Build history of the part. All positions in model axes, mm. Face numbers are marked on the shaded views. A direction names the side the tool comes from. Give positions to 0.01 mm unless a question says otherwise; leave off trailing zeros. Write each loop counter-clockwise with the first axis right and the second up, starting at its lowest first coordinate (ties: lowest second). Pieces come first, ordered by that corner, then holes. Notation, with made-up numbers: (36, -31) -> (41, -31) arc R22 ccw to (41, 6) -> close; hole circle Ø7 at (26.5, 88.25). An arc over 180 degrees is marked (long way). Write item = value, one per line. Start each with the question number.
Q1. Tool access for the marked faces 1 and 2: list every direction of +Z, -Z, +X, -X, +Y, -Y with a clear straight run to the whole face (end or side of a thin tool).
Q2. Wall check: line 1 (X direction, y = 10, z = 3); line 2 (X direction, y = 44, z = 18.5); line 3 (Y direction, x = 140, z = -1.75). Give the ranges that are in metal, low to high.
Q3. Saw through at A-A, the plane x = 31. List the corners of the cut face in (y, z).
Q4. Mould opens along Y. For the marked faces 3, 4, 5 and 6 say: pulls with the +Y half, pulls with the -Y half, needs draft (parallel to the pull), parting line crosses it, or undercut.
Q5. Drop flat-ended pins along their axis: P1, Ø12, axis at x = 107.5, y = 14, coming from the +Z side; P2, Ø1.5, axis at x = 51.5, y = 102.5, coming from the +Z side; P3, Ø1.5, axis at x = 140, y = 117.279, coming from the -Z side. Give the stop position or say it passes through.
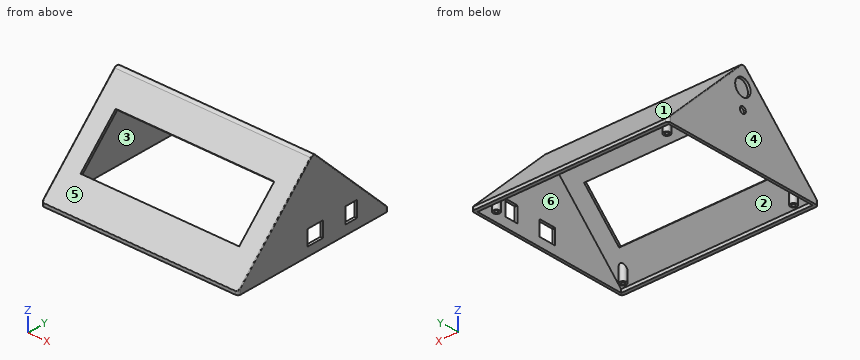
from build123d import *

# Parameters (mm, degrees)
F1_DEPTH  = 150
F2_T      = -2
F4_W      = 121
F4_H      = 42
F5_DEPTH  = 3
F6_R      = 3
F8_R      = 2.5
F8_R_2    = 1.5
F10_R     = 2.5
F10_R_2   = 1.25
F11_REACH = 69.4690374315
F12_W     = 150
F12_H     = 127.2792206136
F12_W_2   = 146
F12_H_2   = 121.6223663641
F13_DEPTH = 2.5
F14_R     = 2.5
F14_R_2   = 1.25
F16_R     = 2
F17_R     = 0.5
F7_W      = 10
F7_H      = 12
F7_W_2    = 13.1
F7_H_2    = 11.7
F18_DEPTH = 3
F19_R     = 0.5
F20_R     = 0.5
F21_R     = 6.5
F22_DEPTH = 2.5
F23_R     = 2.5
F23_R_2   = 1.25
F24_DEPTH = 2.5
F25_R     = 2.5
F26_DEPTH = 1.5
F27_R     = 3


with BuildPart() as f1:
    # F0 (on Right) → F1 (new body)
    with BuildSketch(Plane.YZ):
        Polygon((63.6396103068, 63.6396103068), (0, 0), (127.2792206136, 0), align=None)
    extrude(amount=F1_DEPTH)

    # F2
    f2_openings = [f1.faces().sort_by_distance(p)[0] for p in [
        (75, 63.63961, 0),
    ]]
    offset(amount=F2_T, openings=f2_openings)

    # F4 (on offset) → F5 (cut)
    with BuildSketch(Plane(origin=(0, 0, 0), x_dir=(1, 0, 0), z_dir=(0, -0.7071067812, 0.7071067812))):
        with Locations((75, 45)):
            Rectangle(F4_W, F4_H)
    extrude(amount=-F5_DEPTH, mode=Mode.SUBTRACT)

    # F6
    f6_edges = [f1.edges().sort_by_distance(p)[0] for p in [
        (75, 63.63961, 63.63961),
    ]]
    fillet(f6_edges, radius=F6_R)

    # F8 (on face) → F9 (join, up to the last surface of F1)
    with BuildSketch(Plane(origin=(0, 0, 0), x_dir=(1, 0, 0), z_dir=(0, 0, -1))):
        with Locations((10, -10)):
            Circle(F8_R)
        with Locations((10, -10)):
            Circle(F8_R_2, mode=Mode.SUBTRACT)
    extrude(until=Until.LAST, dir=(0, 0, 1))

    f11_end = Plane(origin=(75.2423938978, 33.320661552, 30.4922344273), x_dir=(0, 0.7071067812, 0.7071067812), z_dir=(0, 0.7071067812, -0.7071067812))
    # F10 (on face) → F11 (join, up to a plane its end follows)
    with BuildSketch(Plane(origin=(0, 0, 0), x_dir=(1, 0, 0), z_dir=(0, 0, -1))):
        with Locations((10, -10)):
            Circle(F10_R)
        with Locations((10, -10)):
            Circle(F10_R_2, mode=Mode.SUBTRACT)
        with Locations((140, -10)):
            Circle(F10_R)
        with Locations((140, -10)):
            Circle(F10_R_2, mode=Mode.SUBTRACT)
    f11_long = extrude(amount=-F11_REACH, mode=Mode.PRIVATE)
    add(split(f11_long, bisect_by=f11_end, keep=Keep.TOP, mode=Mode.PRIVATE))

    # F12 (on face) → F13 (join)
    with BuildSketch(Plane(origin=(0, 0, 0), x_dir=(1, 0, 0), z_dir=(0, 0, -1))):
        with Locations((75, -63.6396103068)):
            Rectangle(F12_W, F12_H)
        with Locations((75, -63.6396103068)):
            Rectangle(F12_W_2, F12_H_2, mode=Mode.SUBTRACT)
    extrude(amount=F13_DEPTH)

    # F14 (on Top) → F15 (join, up to the next surface of F1)
    with BuildSketch(Plane.XY):
        with Locations((140, 117.279)):
            Circle(F14_R)
        with Locations((140, 117.279)):
            Circle(F14_R_2, mode=Mode.SUBTRACT)
        with Locations((10, 117.279)):
            Circle(F14_R)
        with Locations((10, 117.279)):
            Circle(F14_R_2, mode=Mode.SUBTRACT)
    extrude(until=Until.NEXT)

    # F16
    f16_edges = [f1.edges().sort_by_distance(p)[0] for p in [
        (150, 127.279221, -1.25),
        (150, 0, -1.25),
        (0, 0, -1.25),
        (0, 127.279221, -1.25),
    ]]
    fillet(f16_edges, radius=F16_R)

    # F17
    f17_edges = [f1.edges().sort_by_distance(p)[0] for p in [
        (0, 31.759145, 31.759145),
    ]]
    fillet(f17_edges, radius=F17_R)

    # F7 (on face) → F18 (cut)
    with BuildSketch(Plane.YZ.offset(150)):
        with Locations((95.7792206136, 10.65)):
            Rectangle(F7_W, F7_H)
        with Locations((65.3223664939, 10.0139604606)):
            Rectangle(F7_W_2, F7_H_2)
    extrude(amount=-F18_DEPTH, mode=Mode.SUBTRACT)

    # F19
    f19_edges = [f1.edges().sort_by_distance(p)[0] for p in [
        (149, 90.779221, 16.65),
        (149, 100.779221, 16.65),
    ]]
    fillet(f19_edges, radius=F19_R)

    # F20
    f20_edges = [f1.edges().sort_by_distance(p)[0] for p in [
        (149, 71.872366, 15.86396),
        (149, 58.772366, 15.86396),
    ]]
    fillet(f20_edges, radius=F20_R)

    # F21 (on face) → F22 (cut)
    with BuildSketch(Plane(origin=(0, 0, 0), x_dir=(0, -1, 0), z_dir=(-1, 0, 0))):
        with Locations((-64, 47.5)):
            Circle(F21_R)
    extrude(amount=-F22_DEPTH, mode=Mode.SUBTRACT)

    # F23 (on face) → F24 (join)
    with BuildSketch(Plane(origin=(0, 0, 0), x_dir=(1, 0, 0), z_dir=(0, 0, -1))):
        with Locations((10, -10)):
            Circle(F23_R)
        with Locations((10, -10)):
            Circle(F23_R_2, mode=Mode.SUBTRACT)
        with Locations((140, -10)):
            Circle(F23_R)
        with Locations((140, -10)):
            Circle(F23_R_2, mode=Mode.SUBTRACT)
        with Locations((10, -117.279)):
            Circle(F23_R)
        with Locations((10, -117.279)):
            Circle(F23_R_2, mode=Mode.SUBTRACT)
        with Locations((140, -117.279)):
            Circle(F23_R)
        with Locations((140, -117.279)):
            Circle(F23_R_2, mode=Mode.SUBTRACT)
    extrude(amount=F24_DEPTH)

    # F25 (on face) → F26 (cut)
    with BuildSketch(Plane(origin=(0, 0, 0), x_dir=(0, -1, 0), z_dir=(-1, 0, 0))):
        with Locations((-64, 32.5)):
            Circle(F25_R)
    extrude(amount=-F26_DEPTH, mode=Mode.SUBTRACT)

    # F27
    f27_edges = [f1.edges().sort_by_distance(p)[0] for p in [
        (75, 63.63961, 60.811183),
    ]]
    fillet(f27_edges, radius=F27_R)


solid = f1.part
Report:
q1.face_1 = +Z, +X, -X, +Y
q1.face_2 = -Z
q2.line_1 = 0 to 2, 7.5 to 8.75, 11.25 to 12.5, 137.5 to 138.75, 141.25 to 142.5, 148 to 150
q2.line_2 = 0 to 2, 148 to 150
q2.line_3 = 0 to 2.83, 7.5 to 8.75, 11.25 to 12.5, 114.78 to 116.03, 118.53 to 119.78, 124.45 to 127.28
q3.outline = (0, -2.5) -> (2.83, -2.5) -> (2.83, 0) -> (18.38, 15.56) -> (16.97, 16.97) -> (0.15, 0.15) arc R0.5 ccw to (0, -0.21) -> close; (46.67, 46.67) -> (48.08, 45.25) -> (61.52, 58.69) arc R3 cw to (65.76, 58.69) -> (124.45, 0) -> (124.45, -2.5) -> (127.28, -2.5) -> (127.28, -0.21) arc R0.5 ccw to (127.13, 0.15) -> (65.76, 61.52) arc R3 ccw to (61.52, 61.52) -> close
q4.face_3 = undercut
q4.face_4 = needs draft
q4.face_5 = pulls with the -Y half
q4.face_6 = undercut
q5.P1 = 16.97
q5.P2 = 25.53
q5.P3 = 6.42
